from build123d import *

# Parameters (mm, degrees)
F0_W     = 120
F0_H     = 355
F1_DEPTH = 60
F2_W     = 100
F2_H     = 305
F3_DEPTH = 30
F4_T     = -2.5


with BuildPart() as f1:
    # F0 (on Front) → F1 (new body)
    with BuildSketch(Plane.XZ):
        with Locations((60, 177.5)):
            Rectangle(F0_W, F0_H)
    extrude(amount=F1_DEPTH)

    # F2 (on face) → F3 (cut)
    with BuildSketch(Plane.XZ.offset(60)):
        with Locations((120, 177.5)):
            Rectangle(F2_W, F2_H)
    extrude(amount=-F3_DEPTH, mode=Mode.SUBTRACT)

    # F4
    f4_openings = [f1.faces().sort_by_distance(p)[0] for p in [
        (95, -45, 330),
        (70, -45, 177.5),
        (95, -30, 177.5),
        (95, -45, 25),
    ]]
    offset(amount=F4_T, openings=f4_openings)


solid = f1.part
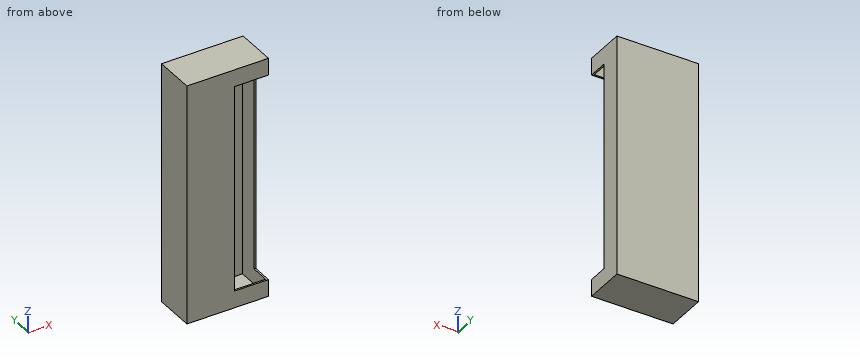
Design review of the part built by this model. Coordinates are the model's own, in mm. Give positions to 0.01 mm unless a question says otherwise; leave off trailing zeros. Loops run counter-clockwise (first coordinate to the right, second up) from the corner with the lowest first, then second, coordinate; pieces in that order, holes last. Notation, with made-up numbers: M -38.5,-24.75 L 19.5,-24.75 A24 cw 19.5,-13.75 Z; hole C 39.5,53.25 d10. An arc over 180 degrees is marked long. Answer as a JSON object with one key per item and string values.
Item 1: We need section D-D (x = 84). State the section outline as (y, z) points, and give its area (3 significant figures).
Output values:
{"outline": "M -60,0 L 0,0 L 0,355 L -60,355 L -60,330 L -57.5,330 L -57.5,352.5 L -2.5,352.5 L -2.5,2.5 L -57.5,2.5 L -57.5,25 L -60,25 Z", "area": "1,290 mm2"}
Item 2: For P1, Ø10, axis at y = -44, z = 151, coming from the +X side; P2, Ø1.2, axis at x = 118, z = 192, coming from the -Y side; P3, Ø1.2, axis at y = -59.5, z = 156, coming from the +X side, all flat-tipped, find the tip position at first contact; note any pin that passes through.
Output values:
{"P1": "stops at x = 2.5", "P2": "stops at y = -30", "P3": "stops at x = 70"}
Item 3: We need section A-A (x = 45.5). State the section outline as (y, z) points.
Output values:
{"outline": "M -60,0 L 0,0 L 0,355 L -60,355 Z; hole M -57.5,2.5 L -2.5,2.5 L -2.5,352.5 L -57.5,352.5 Z"}
Item 4: Wall thickness on line 1 along X through (y, z) = (-10, 55); line 2 along Z through (x, y) = (28.5, -15.5); line 3 along Y through (x, z) = (17.5, 191.5): over which ranges is each line inside the solid? List them lowest first.
Output values:
{"line 1": "x = 0 to 2.5, 117.5 to 120", "line 2": "z = 0 to 2.5, 352.5 to 355", "line 3": "y = -60 to -57.5, -2.5 to 0"}
Item 5: We need section C-C (z = 85). State the section outline as (x, y) points, and give its area (3 significant figures).
Output values:
{"outline": "M 0,-60 L 70,-60 L 70,-57.5 L 2.5,-57.5 L 2.5,-2.5 L 117.5,-2.5 L 117.5,-30 L 120,-30 L 120,0 L 0,0 Z", "area": "681 mm2"}
Item 6: We need section B-B (y = -14). State the section outline as (x, z) points.
Output values:
{"outline": "M 0,0 L 120,0 L 120,355 L 0,355 Z; hole M 2.5,2.5 L 117.5,2.5 L 117.5,352.5 L 2.5,352.5 Z"}
